Here's how the part is built. I have some questions about the finished solid (model axes, mm). Give positions to 0.01 mm unless a question says otherwise; leave off trailing zeros. Loops run counter-clockwise (first coordinate to the right, second up) from the corner with the lowest first, then second, coordinate; pieces in that order, holes last. Notation, with made-up numbers: (1, 18) -> (10, 18) arc R13 cw to (10, 31) -> close; hole circle Ø3 at (75.5, 72.5). An arc over 180 degrees is marked (long way). Answer in a Markdown table with one row per item. Add a question column.
Item 1: For P1, Ø1.5, axis at x = -93.5, y = 2.5, coming from the -Z side; P2, Ø1.5, axis at x = -94.5, y = 3.5, coming from the +Z side; P3, Ø3, axis at x = -103, z = -15.5, coming from the +Y side; P4, Ø2, axis at y = 1.5, z = -65.5, coming from the -X side, each with a flat end and sliding along its axis, tell me the tip position at first contact or that it passes through.
Item 2: If we section it at C-C (x = -56.5): Write out the boundary of the cut face in (y, z).
Item 3: If we section it at B-B (y = 2.9): Give the number of separate pieces and of enclosed holes in the cut face, then the cut area to 3 significant figures.
Item 4: If we section it at D-D (z = -71.5): Write out the boundary of the cut face in (x, y).
Item 5: If we section it at A-A (z = -7): Write out the boundary of the cut face in (x, y).
Item 6: If I drill on line 1 (X direction, y = 3.4, z = 0); line 2 (Z direction, x = 20.5, y = 1.9); line 3 (X direction, y = 1.95, z = 15.5), over which ranges is the centre line in solid material (lowest first)?
```python
from build123d import *

# Parameters (mm, degrees)
SKETCH2_R           = 1.65
SKETCH2_R_2         = 2.25
SKETCH2_R_3         = 15
SKETCH2_R_4         = 2.75
SKETCH2_R_5         = 4.25
BOSS_EXTRUDE3_DEPTH = 5


with BuildPart() as part:
    # Sketch2 → Boss-Extrude3 (new body)
    with BuildSketch(Plane(origin=(0, 0, 0), x_dir=(1, 0, 0), z_dir=(0, 1, 0))):
        with BuildLine():
            Line((-84.557672626, 22.5), (-110, 22.5))
            Line((-110, 22.5), (-110, -22.5))
            Line((-110, -22.5), (-84.557672626, -22.5))
            ThreePointArc((-84.557672626, -22.5), (87.5, 0), (-84.557672626, 22.5))
        make_face()
        with Locations((-103, -15.5)):
            Circle(SKETCH2_R, mode=Mode.SUBTRACT)
        with Locations((-72, -15.5)):
            Circle(SKETCH2_R, mode=Mode.SUBTRACT)
        with Locations((-20.5, -57.830207885)):
            Circle(SKETCH2_R_2, mode=Mode.SUBTRACT)
        with Locations((-20.5, -37.830207885)):
            Circle(SKETCH2_R_2, mode=Mode.SUBTRACT)
        with Locations((20.5, -37.830207885)):
            Circle(SKETCH2_R_2, mode=Mode.SUBTRACT)
        with Locations((-87.5, 0)):
            Circle(SKETCH2_R_3, mode=Mode.SUBTRACT)
        with Locations((-103, 15.5)):
            Circle(SKETCH2_R, mode=Mode.SUBTRACT)
        with Locations((-72, 15.5)):
            Circle(SKETCH2_R, mode=Mode.SUBTRACT)
        with Locations((-18.25, 0)):
            Circle(SKETCH2_R_4, mode=Mode.SUBTRACT)
        Circle(SKETCH2_R_5, mode=Mode.SUBTRACT)
        with Locations((18.25, 0)):
            Circle(SKETCH2_R_4, mode=Mode.SUBTRACT)
        with Locations((-20.5, 37.830207885)):
            Circle(SKETCH2_R_2, mode=Mode.SUBTRACT)
        with Locations((-20.5, 57.830207885)):
            Circle(SKETCH2_R_2, mode=Mode.SUBTRACT)
        with Locations((20.5, 37.830207885)):
            Circle(SKETCH2_R_2, mode=Mode.SUBTRACT)
        with Locations((20.5, 57.830207885)):
            Circle(SKETCH2_R_2, mode=Mode.SUBTRACT)
        with Locations((20.5, -57.830207885)):
            Circle(SKETCH2_R_2, mode=Mode.SUBTRACT)
    extrude(amount=BOSS_EXTRUDE3_DEPTH)


solid = part.part
```
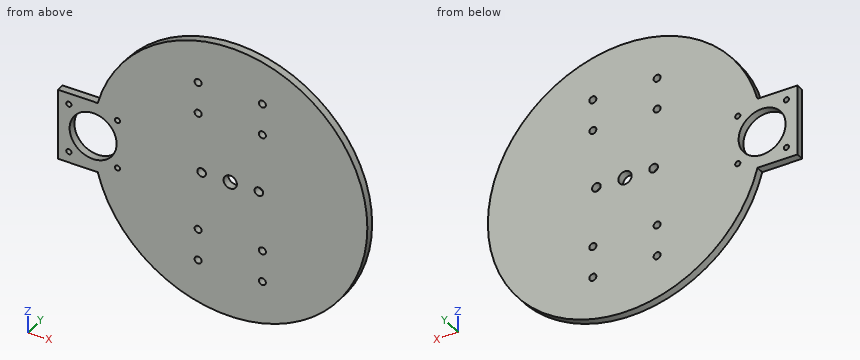
Recorded:
| question | item | result |
|---|---|---|
| 1 | P1 | stops at z = -22.5 |
| 1 | P2 | stops at z = 22.5 |
| 1 | P3 | passes through |
| 1 | P4 | stops at x = -59.13 |
| 2 | outline | (0, -66.81) -> (5, -66.81) -> (5, 66.81) -> (0, 66.81) -> close |
| 3 | separate pieces | 1 |
| 3 | enclosed holes | 16 |
| 3 | area | 24,100 mm^2 |
| 4 | outline | (-50.44, 0) -> (50.44, 0) -> (50.44, 5) -> (-50.44, 5) -> close |
| 5 | outline | (-110, 0) -> (-100.77, 0) -> (-100.77, 5) -> (-110, 5) -> close; (-74.23, 0) -> (87.22, 0) -> (87.22, 5) -> (-74.23, 5) -> close |
| 6 | line 1 | x = -110 to -102.5, -72.5 to -21, -15.5 to -4.25, 4.25 to 15.5, 21 to 87.5 |
| 6 | line 2 | z = -85.06 to -60.08, -55.58 to -40.08, -35.58 to -1.58, 1.58 to 35.58, 40.08 to 55.58, 60.08 to 85.06 |
| 6 | line 3 | x = -110 to -104.65, -101.35 to -73.65, -70.35 to 86.12 |
